Autodesk Fusion 360 part; units mm, degrees
sketch "PCB" plane through (0, 0, 0) normal (0, 0, 1) x (1, 0, 0)
  line L0 (-71.6509, 41.0939) -> (266.3491, 41.0939)
  line L1 (266.3491, 41.0939) -> (266.3491, -61.9061)
  line L2 (266.3491, -61.9061) -> (-71.6509, -61.9061)
  line L3 (-71.6509, -61.9061) -> (-71.6509, 41.0939)
  circle A0 centre (-45.1809, -36.3161) radius 1.6
  circle A1 centre (-14.4909, 13.0239) radius 1.6
  circle A2 centre (115.9291, -47.8061) radius 1.6
  circle A3 centre (243.8291, -38.8761) radius 1.6
  circle A4 centre (241.5491, 15.1939) radius 1.6
  line L4 (-60.6509, 41.0939) -> (-51.6509, 41.0939)
  line L5 (-51.6509, 41.0939) -> (-51.6509, 34)
  line L6 (-51.6509, 34) -> (-60.6509, 34)
  line L7 (-60.6509, 34) -> (-60.6509, 41.0939)
  point P0 (-45.4739, -36.5361)
  point P1 (-40.6298, 20.2839)
  dimension "d1" = 338
  dimension "d2" = 103
  dimension "d3" = 3.2
  dimension "d4" = 25.59
  dimension "d5" = 26.47
  dimension "d6" = 3.2
  dimension "d7" = 28.07
  dimension "d8" = 57.16
  dimension "d9" = 3.2
  dimension "d10" = 14.1
  dimension "d11" = 150.42
  dimension "d12" = 3.2
  dimension "d13" = 22.52
  dimension "d14" = 23.03
  dimension "d15" = 3.2
  dimension "d16" = 24.8
  dimension "d17" = 25.9
  dimension "d32" = 11
  dimension "d33" = 20
sketch "Sketch2" plane through (0, 0, 0) normal (0, 0, 1) x (1, 0, 0)
  line L0 (-76.6509, 46.0939) -> (271.3491, 46.0939)
  line L1 (271.3491, 46.0939) -> (271.3491, -66.9061)
  line L2 (271.3491, -66.9061) -> (-76.6509, -66.9061)
  line L3 (-76.6509, -66.9061) -> (-76.6509, 46.0939)
  line L4 (-71.6509, 41.0939) -> (266.3491, 41.0939)
  line L5 (-71.6509, -61.9061) -> (-71.6509, 41.0939)
  line L6 (266.3491, -61.9061) -> (-71.6509, -61.9061)
  line L7 (266.3491, 41.0939) -> (266.3491, -61.9061)
  line L8 (-72.6509, 42.0939) -> (267.3491, 42.0939)
  line L9 (267.3491, 42.0939) -> (267.3491, -62.9061)
  line L10 (267.3491, -62.9061) -> (-72.6509, -62.9061)
  line L11 (-72.6509, -62.9061) -> (-72.6509, 42.0939)
  line L12 (-51.6509, 46.0939) -> (-51.6509, 39)
  line L13 (-60.6509, 39) -> (-60.6509, 46.0939)
  line L14 (-51.6509, 39) -> (-60.6509, 39)
  dimension "d18" = 5
  dimension "d19" = 5
  dimension "d20" = 5
  dimension "d21" = 5
  dimension "d24" = 4
  dimension "d25" = 4
  dimension "d26" = 4
  dimension "d27" = 4
extrude "Extrude1" add sketch "Sketch2" along normal blind 5 contours L4 L5 L6 L7 L12 L13 L14 | L4 L12 L13 L14
extrude "Extrude2" add sketch "Sketch2" along normal blind 5 contours L4 L5 L6 L7 L8 L9 L10 L11 L12 L13 | L4 L8 L12 L13
extrude "Extrude3" add sketch "Sketch2" along normal blind 13 contours L0 L1 L2 L3 L8 L9 L10 L11 L12 L13 | L0 L8 L12 L13
sketch "Sketch3" plane through (0, 0, 13) normal (0, 0, 1) x (-1, 0, 0)
  line L0 (-267.3491, 62.9061) -> (72.6509, 62.9061)
  line L1 (72.6509, 62.9061) -> (72.6509, -42.0939)
  line L2 (72.6509, -42.0939) -> (-267.3491, -42.0939)
  line L3 (-267.3491, -42.0939) -> (-267.3491, 62.9061)
  line L4 (76.6509, 66.9061) -> (-271.3491, 66.9061)
  line L5 (-271.3491, 66.9061) -> (-271.3491, -46.0939)
  line L6 (-271.3491, -46.0939) -> (76.6509, -46.0939)
  line L7 (76.6509, -46.0939) -> (76.6509, 66.9061)
  line L8 (65.1904, -46.0939) -> (45.472, -46.0939)
  line L9 (45.472, -46.0939) -> (45.472, -42.0939)
  line L10 (45.472, -42.0939) -> (65.1904, -42.0939)
  line L11 (65.1904, -42.0939) -> (65.1904, -46.0939)
extrude "Extrude4" cut sketch "Sketch3" against normal blind 5 contours L2 L6 L8 L9 L10 L11
sketch "HOLWS" plane through (0, 0, 5) normal (0, 0, 1) x (-1, 0, 0)
  line L0 (72.6509, 62.9061) -> (-267.3491, 62.9061)
  line L1 (-267.3491, 62.9061) -> (-267.3491, -42.0939)
  line L2 (-267.3491, -42.0939) -> (72.6509, -42.0939)
  line L3 (72.6509, -42.0939) -> (72.6509, 62.9061)
  circle A0 centre (14.5, -13) radius 2.15
  circle A1 centre (46.6409, 51.0461) radius 2.15
  circle A2 centre (-115.929, 47.8061) radius 2.15
  circle A3 centre (-243.8291, 38.876) radius 2.15
  circle A4 centre (-241.5493, -15.1935) radius 2.15
  dimension "d48" = 4.3
  dimension "d49" = 4.3
  dimension "d50" = 4.3
  dimension "d51" = 4.3
  dimension "d52" = 4.3
  dimension "d57" = 26.01
  dimension "d58" = 11.86
fillet "Fillet1" radius 1 1 edges at (-76.6509, -66.9061, 6.5)
fillet "Fillet2" radius 1 1 edges at (-76.6509, 46.0939, 6.5)
fillet "Fillet3" radius 1 1 edges at (271.3491, -66.9061, 6.5)
fillet "Fillet4" radius 1 1 edges at (271.3491, 46.0939, 6.5)
sketch "Sketch5" plane through (0, 0, 0) normal (0, 0, 1) x (1, 0, 0)
  line L0 (256.3491, 36.2293) -> (-61.6509, 36.2293)
  line L1 (-61.6509, 36.2293) -> (-61.6509, 24.2668)
  line L2 (-61.6509, 24.2668) -> (256.3491, 24.2668)
  line L3 (256.3491, 24.2668) -> (256.3491, 36.2293)
  line L4 (-71.6509, -61.9061) -> (-71.6509, 41.0939)
  line L5 (266.3491, 41.0939) -> (266.3491, -61.9061)
  dimension "d44" = 10
  dimension "d45" = 10
extrude "Extrude5" add sketch "Sketch5" against normal blind 3
extrude "Extrude6" cut sketch "HOLWS" against normal blind 3.2 contours A0 | A1 | A2 | A3 | A4
chamfer "Chamfer1" distance 0.35 angle 45 1 edges at (-12.4955, 12.2225, 5)
chamfer "Chamfer2" distance 0.35 angle 45 4 edges at (-44.6364, -51.8236, 5) (117.9335, -48.5836, 5) (243.5538, 14.416, 5) (245.8336, -39.6534, 5)
move_body "Move1" bodies 1 to x (1, 0, 0) y (0, 1, 0) z (0, 0, 1) at (60, 0, 0)
move_body "Move2" bodies 1 to x (1, 0, 0) y (0, 1, 0) z (0, 0, 1) at (0, -5, 0)
move_body "Move3" bodies 1 to x (1, 0, 0) y (0, 1, 0) z (0, 0, 1) at (-60, 5, 0)
sketch "Sketch6" plane through (0, 0, 1.8) normal (0, 0, 1) x (-1, 0, 0)
  circle A0 centre (14.5, -13) radius 2.15
Verification items for the finished model (mm, model axes). A direction names the side the tool comes from. Coordinates: 2 decimals unless noted, no trailing zeros. Loops run counter-clockwise (first coordinate to the right, second up) from the corner with the lowest first, then second, coordinate; pieces in that order, holes last. Notation, with made-up numbers: M 78.25,15.25 L 127.25,15.25 A33 ccw 127.25,53.25 Z; hole C 62.25,45 d6. An arc over 180 degrees is marked long. One line per item, written item: value.
1. Set-up check for faces 4 (the flat face through (100, -62.906, 9)), 5 (the flat face through (97, -65, 13)): record each of +Z, -Z, +X, -X, +Y, -Y from which the full face is reachable in a straight line by a thin tool's end or side.
Answers follow:
face 4: +Z
face 5: +Z, +X, -X, +Y, -Y
2. Material ranges on line 1 along X through (y, z) = (19, 12); line 2 along X through (y, z) = (13, 3.05); line 3 along Y through (x, z) = (71, 10), recorded low to high. Write a range as from..to.
Answers follow:
line 1: -76.65..-72.65, 267.35..271.35
line 2: -76.65..-16.65, -12.35..271.35
line 3: -66.91..-62.91, 42.09..46.09
3. Gauge pin test, flat ends, axial feed: P1, Ø1, axis at x = -1.5, y = 22, coming from the +Z side; P2, Ø1.5, axis at x = 74.5, z = -1, coming from the -Y side; P3, Ø1.5, axis at x = 55.5, z = -1, coming from the +Y side. Record the tip position at first contact, or that the pin passes through.
Answers follow:
P1: z = 5
P2: y = 24.27
P3: y = 36.23
4. Section check B-B on y = -7. Record the cut outline in (x, z), plus the area to 3 significant figures.
Answers follow:
outline: M -76.65,0 L 271.35,0 L 271.35,13 L 267.35,13 L 267.35,5 L -72.65,5 L -72.65,13 L -76.65,13 Z
area: 1,800 mm^2
5. Section check A-A on x = 32. Record the cut outline in (y, z), plus the area to 3 significant figures.
Answers follow:
outline: M -66.91,0 L 24.27,0 L 24.27,-3 L 36.23,-3 L 36.23,0 L 46.09,0 L 46.09,13 L 42.09,13 L 42.09,5 L -62.91,5 L -62.91,13 L -66.91,13 Z
area: 665 mm^2
6. Mould release check, pull along Y, two halves, no side actions. Record for faces 1 (the flat face through (-76.651, -11, 6)), 2 (the flat face through (95, 42.094, 9)), 3 (the flat face through (100, -66.906, 6)): pulls with the +Y half, pulls with the -Y half, needs draft (parallel to the pull), parting line crosses it, or undercut.
Answers follow:
face 1: needs draft
face 2: undercut
face 3: pulls with the -Y half
